```python
from build123d import *

# Parameters (mm, degrees)
SKETCH2_R           = 10
BOSS_EXTRUDE1_DEPTH = 8
SKETCH3_R           = 10
BOSS_EXTRUDE2_DEPTH = 8
SKETCH4_R           = 10
BOSS_EXTRUDE3_DEPTH = 8
FILLET1_R           = 5


with BuildPart() as part:
    # Sketch2 → Boss-Extrude1 (new body)
    with BuildSketch(Plane(origin=(0, 0, 0), x_dir=(1, 0, 0), z_dir=(0, 1, 0))):
        with BuildLine():
            Line((0, 0), (0, 89))
            Line((0, 89), (57, 89))
            Line((57, 89), (57, 79.5))
            ThreePointArc((57, 79.5), (60.807611845, 70.307611845), (70, 66.5))
            Line((70, 66.5), (111, 66.5))
            ThreePointArc((111, 66.5), (133, 44.5), (111, 22.5))
            Line((111, 22.5), (70, 22.5))
            ThreePointArc((70, 22.5), (60.807611845, 18.692388155), (57, 9.5))
            Line((57, 9.5), (57, 0))
            Line((57, 0), (0, 0))
        make_face()
        with Locations((73, 44.5)):
            Circle(SKETCH2_R, mode=Mode.SUBTRACT)
        with Locations((111, 44.5)):
            Circle(SKETCH2_R, mode=Mode.SUBTRACT)
    extrude(amount=BOSS_EXTRUDE1_DEPTH)

    # Sketch3 → Boss-Extrude2 (add)
    with BuildSketch(Plane.XY):
        with BuildLine():
            Line((0, 0), (57, 0))
            Line((57, 0), (57, 36.5))
            ThreePointArc((57, 36.5), (28.5, 65), (0, 36.5))
            Line((0, 36.5), (0, 0))
        make_face()
        with Locations((28.5, 36.5)):
            Circle(SKETCH3_R, mode=Mode.SUBTRACT)
    extrude(amount=-BOSS_EXTRUDE2_DEPTH)

    # Sketch4 → Boss-Extrude3 (add)
    with BuildSketch(Plane(origin=(0, 0, -89), x_dir=(-1, 0, 0), z_dir=(0, 0, -1))):
        with BuildLine():
            Line((-57, 8), (0, 8))
            Line((0, 8), (0, 36.5))
            ThreePointArc((0, 36.5), (-28.5, 65), (-57, 36.5))
            Line((-57, 36.5), (-57, 8))
        make_face()
        with Locations((-28.5, 36.5)):
            Circle(SKETCH4_R, mode=Mode.SUBTRACT)
    extrude(amount=-BOSS_EXTRUDE3_DEPTH)

    # Fillet1
    fillet1_edges = [part.edges().sort_by_distance(p)[0] for p in [
        (28.5, 8, -8),
        (28.5, 8, -81),
    ]]
    fillet(fillet1_edges, radius=FILLET1_R)


solid = part.part
```
The model under review builds one solid part; all positions refer to its coordinate system, in mm. A direction names the side the tool comes from. Give positions to 0.01 mm unless a question says otherwise; leave off trailing zeros. Write each loop counter-clockwise with the first axis right and the second up, starting at its lowest first coordinate (ties: lowest second). Pieces come first, ordered by that corner, then holes. Notation, with made-up numbers: M 21,18.5 L 72,18.5 A17 cw 72,29.5 Z; hole C -35,49 d2. An arc over 180 degrees is marked long. Write item = value, one per line. Start each with the question number.
Q1. Mouldability with a two-part tool opening along Z and no side actions: class faces 5 (the face through (30.67, 26.74, -85.06)), 6 (the face through (28, 10, -9)), 7 (the face through (90, 4, -66.5)) as released by +Z, released by -Z, zero draft, split by the parting line, or undercut.
Q2. Machinability: for faces 1 (the face through (34.4, 45.1, -8)), 2 (the face through (53, 0, -45)), 3 (the face through (91, 4, -22.5)), 4 (the face through (57, 19, -84)), which of the approach directions +Z, -Z, +X, -X, +Y, -Y give a long, thin tool a straight path to every point of the face, cutting with its end or side? Answer none if there is none.
Q3. For line 1 (Z direction, x = 111, y = 2.75); line 2 (Y direction, x = 28, z = -86); line 3 (X direction, y = 36, z = -2), list the stretches that pass through material, from the lowest coordinate up.
Q4. Clearance check with flat-ended pins moving along their axes: pin 1 (2.5 mm diameter, centred on x = 93.5, y = 2.5, fed in from -Z); pin 2 (12 mm diameter, centred on x = 111, z = -44.5, fed in from -Y); pin 3 (7.5 mm diameter, centred on y = 25.5, z = -5, fed in from +X); pin 4 (9 mm diameter, centred on x = 95.5, y = 5, fed in from +Z). State where each tip first meets the part, or that it passes through.
Q5. We need section A-A (z = -44.5). State the section outline as (x, y) points, plus the area to 3 significant figures.
Q6. We need section B-B (y = 19). State the section outline as (x, z) points, plus the area to 3 significant figures.
Q7. We need section C-C (x = 103). State the section outline as (y, z) points, plus the area to 3 significant figures.
Q8. We need section D-D (y = 30.5). State the section outline as (x, z) points, plus the area to 3 significant figures.
Result set:
q1.face_5 = zero draft
q1.face_6 = undercut
q1.face_7 = released by -Z
q2.face_1 = +X, -X, +Y
q2.face_2 = +Z, -Z, +X, -X, -Y
q2.face_3 = +Z, +X, +Y, -Y
q2.face_4 = -Z, +X, +Y, -Y
q3.line_1 = -66.5 to -54.5, -34.5 to -22.5
q3.line_2 = 0 to 26.51, 46.49 to 65
q3.line_3 = 0 to 18.51, 38.49 to 57
q4.pin_1 = -66.5
q4.pin_2 = through
q4.pin_3 = 57
q4.pin_4 = -22.5
q5.outline = M 0,0 L 63,0 L 63,8 L 0,8 Z; M 83,0 L 101,0 L 101,8 L 83,8 Z; M 121,0 L 133,0 L 133,8 L 121,8 Z
q5.area = 744 mm2
q6.outline = M 0,-89 L 57,-89 L 57,-81 L 0,-81 Z; M 0,-8 L 57,-8 L 57,0 L 0,0 Z
q6.area = 912 mm2
q7.outline = M 0,-66.5 L 8,-66.5 L 8,-50.5 L 0,-50.5 Z; M 0,-38.5 L 8,-38.5 L 8,-22.5 L 0,-22.5 Z
q7.area = 256 mm2
q8.outline = M 0,-89 L 20.5,-89 L 20.5,-81 L 0,-81 Z; M 0,-8 L 20.5,-8 L 20.5,0 L 0,0 Z; M 36.5,-89 L 57,-89 L 57,-81 L 36.5,-81 Z; M 36.5,-8 L 57,-8 L 57,0 L 36.5,0 Z
q8.area = 656 mm2
